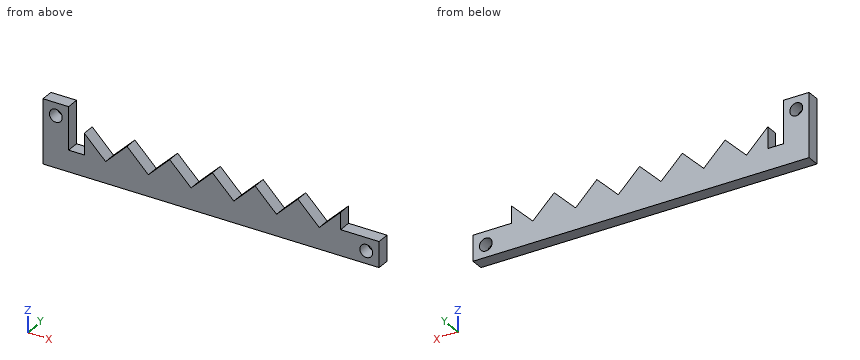
```python
from build123d import *

# Parameters (mm, degrees)
SKETCH1_R           = 1.5
BOSS_EXTRUDE1_DEPTH = 3


with BuildPart() as part:
    # Sketch1 → Boss-Extrude1 (new body)
    with BuildSketch(Plane(origin=(0, 0, 0), x_dir=(1, 0, 0), z_dir=(0, 1, 0))):
        Polygon((1.765756862, 34.483992996), (6.765756862, 39.483992996), (11.765756862, 34.483992996), (16.765756862, 39.483992996), (21.765756862, 34.483992996), (26.765756862, 39.483992996), (31.765756862, 34.483992996), (36.765756862, 39.483992996), (41.765756862, 34.483992996), (46.765756862, 39.483992996), (51.765756862, 34.483992996), (56.765756862, 39.483992996), (61.765756862, 34.483992996), (61.765756862, 38.483992996), (70.765756862, 38.483992996), (70.765756862, 44.483992996), (1, 44.483992996), (-5.848815236, 44.483992996), (-7.891171506, 44.483992996), (-7.891171506, 29.483992996), (-1.891171506, 29.483992996), (-1.891171506, 39.483992996), (1.765756862, 39.483992996), align=None)
        with Locations((-4.891171506, 32.483992996)):
            Circle(SKETCH1_R, mode=Mode.SUBTRACT)
        with Locations((67.765756862, 41.557757711)):
            Circle(SKETCH1_R, mode=Mode.SUBTRACT)
    extrude(amount=BOSS_EXTRUDE1_DEPTH)


solid = part.part
```
Can you work these out from the model? Positions are in its coordinate system, mm. Give positions to 0.01 mm unless a question says otherwise; leave off trailing zeros. Loops run counter-clockwise (first coordinate to the right, second up) from the corner with the lowest first, then second, coordinate; pieces in that order, holes last. Notation, with made-up numbers: M 0,-26.75 L 7,-26.75 A22 cw 7,-0.75 Z; hole C 56.25,78 d10. An arc over 180 degrees is marked long. Answer in a Markdown table with one row per item.
1. Suppose I cut it at C-C on x = 15. Write out the boundary of the cut face in (y, z), plus the area to 3 significant figures.
Taken from the geometry:
| item | result |
|---|---|
| outline | M 0,-44.48 L 3,-44.48 L 3,-37.72 L 0,-37.72 Z |
| area | 20.3 mm² |
2. Suppose I cut it at A-A on z = -40.75. Write out the boundary of the cut face in (x, y).
Taken from the geometry:
| item | result |
|---|---|
| outline | M -7.89,0 L 66.5,0 L 66.5,3 L -7.89,3 Z; M 69.03,0 L 70.77,0 L 70.77,3 L 69.03,3 Z |
3. If I drill on line 1 along X through (y, z) = (2.5, -40.25); line 2 along X through (y, z) = (2.2, -33.25); line 3 along X through (y, z) = (0.75, -34.25), over which ranges is the centre line in solid material (lowest first)?
Taken from the geometry:
| item | result |
|---|---|
| line 1 | x = -7.89 to 67.03, 68.5 to 70.77 |
| line 2 | x = -7.89 to -6.18, -3.6 to -1.89 |
| line 3 | x = -7.89 to -1.89 |
4. For pin 1 Ø1.5 at (y, z) = (1.5, -36) entering from +X; pin 2 Ø2.5 at (x, z) = (67.77, -41.56) entering from -Y; pin 3 Ø0.9 at (x, y) = (-1, 1) entering from +Z, each with a flat end and sliding along its axis, tell me the tip position at first contact or that it passes through.
Taken from the geometry:
| item | result |
|---|---|
| pin 1 | stops at x = 61.77 |
| pin 2 | passes through |
| pin 3 | stops at z = -39.48 |
5. Suppose I cut it at B-B on y = 1.25. Write out the boundary of the cut face in (x, z).
Taken from the geometry:
| item | result |
|---|---|
| outline | M -7.89,-44.48 L 70.77,-44.48 L 70.77,-38.48 L 61.77,-38.48 L 61.77,-34.48 L 56.77,-39.48 L 51.77,-34.48 L 46.77,-39.48 L 41.77,-34.48 L 36.77,-39.48 L 31.77,-34.48 L 26.77,-39.48 L 21.77,-34.48 L 16.77,-39.48 L 11.77,-34.48 L 6.77,-39.48 L 1.77,-34.48 L 1.77,-39.48 L -1.89,-39.48 L -1.89,-29.48 L -7.89,-29.48 Z; hole C -4.89,-32.48 d3; hole C 67.77,-41.56 d3 |
6. Suppose I cut it at D-D on x = 4. Write out the boundary of the cut face in (y, z).
Taken from the geometry:
| item | result |
|---|---|
| outline | M 0,-44.48 L 3,-44.48 L 3,-36.72 L 0,-36.72 Z |
